```python
from build123d import *

# Parameters (mm, degrees)
F0_R      = 30
F0_W      = 5
F0_H      = 5
F3_DEPTH  = 3.5
F1_R      = 1.875
F4_DEPTH  = 25
F2_R      = 1.875
F5_DEPTH  = 25
F6_R      = 2
F7_R      = 3
F8_DEPTH  = 30
F10_R     = 1.575
F11_DEPTH = 7


with BuildPart() as f3:
    # F0 (on Top) → F3 (new body)
    with BuildSketch(Plane.XY):
        Polygon((69.5, -35), (74, -35), (74, 35), (69.5, 35), (64.5, 35), (-64.5, 35), (-69.5, 35), (-74, 35), (-74, -35), (-69.5, -35), (-69.5, -43), (-64.5, -43), (-64.5, -35), (64.5, -35), (64.5, -43), (69.5, -43), align=None)
        with Locations((-37, 0)):
            Circle(F0_R, mode=Mode.SUBTRACT)
        with Locations((37, 0)):
            Circle(F0_R, mode=Mode.SUBTRACT)
        with Locations((67, 37.5)):
            Rectangle(F0_W, F0_H)
        with Locations((-67, 37.5)):
            Rectangle(F0_W, F0_H)
    extrude(amount=F3_DEPTH)

    # F1 (on face) → F4 (cut)
    with BuildSketch(Plane.XY):
        with Locations((-62.19, 25.19)):
            Circle(F1_R)
        with Locations((-11.81, 25.19)):
            Circle(F1_R)
        with Locations((-62.19, -25.19)):
            Circle(F1_R)
        with Locations((-11.81, -25.19)):
            Circle(F1_R)
    extrude(amount=F4_DEPTH, mode=Mode.SUBTRACT)

    # F2 (on Top) → F5 (cut)
    with BuildSketch(Plane.XY):
        with Locations((11.81, 25.19)):
            Circle(F2_R)
        with Locations((11.81, -25.19)):
            Circle(F2_R)
        with Locations((62.19, 25.19)):
            Circle(F2_R)
        with Locations((62.19, -25.19)):
            Circle(F2_R)
    extrude(amount=F5_DEPTH, mode=Mode.SUBTRACT)

    # F6
    f6_edges = [f3.edges().sort_by_distance(p)[0] for p in [
        (-67, 0, 3.5),
        (7, 0, 3.5),
    ]]
    fillet(f6_edges, radius=F6_R)

    # F7 (on Top) → F8 (join)
    with BuildSketch(Plane.XY):
        with Locations((-67, -40.5)):
            Circle(F7_R)
        with Locations((67, -40.5)):
            Circle(F7_R)
        with Locations((-67, 34.5)):
            Circle(F7_R)
        with Locations((67, 34.5)):
            Circle(F7_R)
    extrude(amount=-F8_DEPTH)

    # F10 (on offset) → F11 (cut)
    with BuildSketch(Plane.XY.offset(-30)):
        with Locations((-67, -40.5)):
            Circle(F10_R)
        with Locations((-67, 34.5)):
            Circle(F10_R)
        with Locations((67, -40.5)):
            Circle(F10_R)
        with Locations((67, 34.5)):
            Circle(F10_R)
    extrude(amount=F11_DEPTH, mode=Mode.SUBTRACT)


solid = f3.part
```
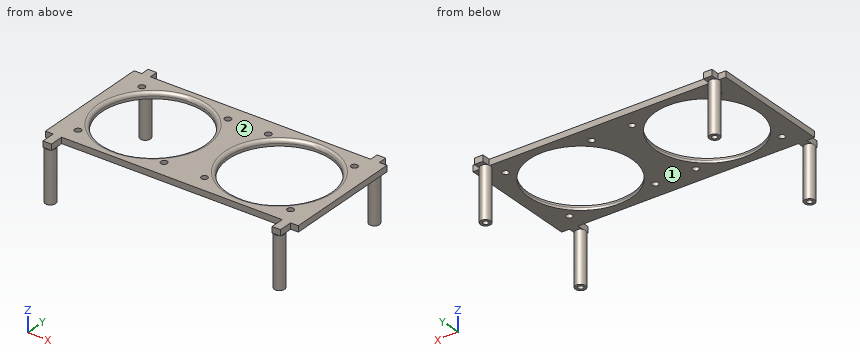
The listing builds one solid part. Answer for the finished solid, in the listing's coordinates (mm). Face numbers are marked on the shaded views. Coordinates: 2 decimals unless noted, no trailing zeros. Order: outer loops, then holes, each group sorted by start corner. A loop starts at its lowest first (then second) coordinate and runs counter-clockwise, first axis right, second up. Notation, with made-up numbers: M 39,7.25 L 62,7.25 A11 cw 62,20.25 Z; hole C -11,-3.75 d8. An arc over 180 degrees is marked long. Answer as a JSON object with one key per item and string values. Group by question number.
1. Section C-C on z = -8.5 is taken. Write down the section's boundary in (x, y), then the cut area to 3 significant figures.
2. Section B-B on y = 0 is taken. Write down the section's boundary in (x, z).
3. Flat-ended cylindrical pins translate along their axes: P1, Ø4, axis at x = -70.5, z = 2, coming from the -Y side; P2, Ø12, axis at x = -30.5, z = -0.5, coming from the -Y side; P3, Ø3, axis at y = 37, z = 1.5, coming from the -X side. Find the tip coordinate at first contact, or state that the pin passes through.
4. Straight lines are drawn through the part: line 1 (Y direction, x = 67, z = -25.5) (3 decimals); line 2 (X direction, y = -38.5, z = 2.5); line 3 (Y direction, x = 11, z = 1). For each, find the intervals that lie inside material, in ascending order.
5. Determine the mould class of the marked faces 1 and 2 for opening direction Y: released by +Y, released by -Y, zero draft, split by the parting line, or undercut.
6. Section D-D on x = -1.5 is taken. Write down the section's boundary in (y, z).
7. Section A-A on x = 37 is taken. Write down the section's boundary in (y, z), then the cut area to 3 significant figures.
Values follow:
{
 "1": {"outline": "C -67,-40.5 d6; C -67,34.5 d6; C 67,-40.5 d6; C 67,34.5 d6", "area": "113 mm2"},
 "2": {"outline": "M -74,0 L -67,0 L -67,1.5 A2 ccw -69,3.5 L -74,3.5 Z; M -7,0 L 7,0 L 7,1.5 A2 ccw 5,3.5 L -5,3.5 A2 ccw -7,1.5 Z; M 67,0 L 74,0 L 74,3.5 L 69,3.5 A2 ccw 67,1.5 Z"},
 "3": {"P1": "y = -43", "P2": "y = -35", "P3": "x = -69.5"},
 "4": {"line 1": "-43.5 to -42.075, -38.925 to -37.5, 31.5 to 32.925, 36.075 to 37.5", "line 2": "-69.5 to -64.5, 64.5 to 69.5", "line 3": "-35 to -26.88, -23.5 to -14.97, 14.97 to 23.5, 26.88 to 35"},
 "5": {"face 1": "undercut", "face 2": "zero draft"},
 "6": {"outline": "M -35,0 L 35,0 L 35,3.5 L -35,3.5 Z"},
 "7": {"outline": "M -35,0 L -30,0 L -30,1.5 A2 ccw -32,3.5 L -35,3.5 Z; M 30,0 L 35,0 L 35,3.5 L 32,3.5 A2 ccw 30,1.5 Z", "area": "33.3 mm2"}
}
